Autodesk Inventor part; units mm, degrees
ref_plane "YZ Plane" through (0, 0, 0) normal (1, 0, 0) x (0, 1, 0)
ref_plane "XZ Plane" through (0, 0, 0) normal (0, 1, 0) x (-1, 0, 0)
ref_plane "XY Plane" through (0, 0, 0) normal (0, 0, 1) x (1, 0, 0)
sketch "スケッチ1" plane through (0, 0, 0) normal (0, 1, 0) x (-1, 0, 0)
  circle A0 centre (0, 0) radius 3
  dimension "d0" = 6
extrude "押し出し1" add sketch "スケッチ1" along normal mid plane 10
sketch "スケッチ2" plane through (0, 5, 0) normal (0, 1, 0) x (1, 0, 0)
  point P0 (0, 0)
  point P1 (0, 0)
hole "穴1" at (0, 5, 0) direction (0, -1, 0) diameter 2.459 depth 10 countersink diameter 3.4 countersink angle 90
sketch "スケッチ3" plane through (0, -5, 0) normal (0, -1, 0) x (1, 0, 0)
  point P0 (0, 0)
  point P1 (0, 0)
hole "穴2" at (0, -5, 0) direction (0, 1, 0) diameter 2.459 depth 10 countersink diameter 3.4 countersink angle 90
chamfer "面取り1" distance 0.25 angle 45 2 edges at (3, -5, 0) (3, 5, 0)
properties part number "Spacer_M3D6L60" material "アルミニウム 6061"
Model file for the job. Use its own axes, mm. Give positions to 0.01 mm unless a question says otherwise; leave off trailing zeros. Write each loop counter-clockwise with the first axis right and the second up, starting at its lowest first coordinate (ties: lowest second). Pieces come first, ordered by that corner, then holes. Notation, with made-up numbers: (12, -35) - (47, -35) arc R28 cw to (47, -1) - close; hole circle Ø6 at (48, 47.25). An arc over 180 degrees is marked (long way). Answer as CSV lines item,"result".
1. Band-saw the part on C-C (y = 2). Write the cut outline in (x, z), and give its area (3 significant figures).
Responses:
outline,"circle Ø6 at (0, 0); hole circle Ø2.46 at (0, 0)"
area,"23.5 mm2"
2. Pin check, flat tips, straight feed: pin 1 (3 mm diameter, centred on y = 0, z = -2, fed in from +X); pin 2 (2 mm diameter, centred on y = -2.5, z = 2, fed in from +X); pin 3 (1.5 mm diameter, centred on y = 1, z = 1.5, fed in from -X); pin 4 (1.5 mm diameter, centred on x = -1, z = 0.5, fed in from -Y). Stop position of each tip, or through.
Responses:
pin 1,"stops at x = 2.96"
pin 2,"stops at x = 2.83"
pin 3,"stops at x = -2.9"
pin 4,"stops at y = -5"
3. Two-plate mould, pull along X, no slides. Class faces 1 (the face through (3, 0, 0)), 2 (the face through (-2, -5, 0)), 3 (the face through (0.748, -0.063, -0.976)): +X half, -X half, draft (parallel to the pull), parting line (faces both ways), or undercut.
Responses:
face 1,"parting line"
face 2,"draft"
face 3,"undercut"
4. Band-saw the part on B-B (z = 0). Write the cut outline in (x, y).
Responses:
outline,"(-3, -4.75) - (-2.75, -5) - (-1.7, -5) - (-1.23, -4.53) - (-1.23, 4.53) - (-1.7, 5) - (-2.75, 5) - (-3, 4.75) - close; (1.23, -4.53) - (1.7, -5) - (2.75, -5) - (3, -4.75) - (3, 4.75) - (2.75, 5) - (1.7, 5) - (1.23, 4.53) - close"
5. Drill centre lines: L1, parallel to Z at x = 0, y = -2.5; L2, parallel to Z at x = -0.6, y = -4.5; L3, parallel to X at y = -0.5, z = -0.65. Where is each one in solid material? Low to high. Write a range as [from, to].
Responses:
L1,"z = [-3, -1.23], [1.23, 3]"
L2,"z = [-2.94, -1.07], [1.07, 2.94]"
L3,"x = [-2.93, -1.04], [1.04, 2.93]"
6. Band-saw the part on A-A (x = 0). Write the cut outline in (y, z), and give its area (3 significant figures).
Responses:
outline,"(-5, -2.75) - (-4.75, -3) - (4.75, -3) - (5, -2.75) - (5, -1.7) - (4.53, -1.23) - (-4.53, -1.23) - (-5, -1.7) - close; (-5, 1.7) - (-4.53, 1.23) - (4.53, 1.23) - (5, 1.7) - (5, 2.75) - (4.75, 3) - (-4.75, 3) - (-5, 2.75) - close"
area,"34.8 mm2"
